```python
from build123d import *

# Parameters (mm, degrees)
F0_W     = 55
F0_H     = 100
F0_R     = 1.55
F0_R_2   = 3.05
F1_DEPTH = 5
F2_SIZE  = 1.5


with BuildPart() as f1:
    # F0 (on Top) → F1 (new body)
    with BuildSketch(Plane.XY):
        with Locations((0, 22.5)):
            Rectangle(F0_W, F0_H)
        with Locations((-20, -22.5)):
            Circle(F0_R, mode=Mode.SUBTRACT)
        with Locations((20, -22.5)):
            Circle(F0_R, mode=Mode.SUBTRACT)
        with Locations((-20, 22.5)):
            Circle(F0_R, mode=Mode.SUBTRACT)
        with Locations((20, 22.5)):
            Circle(F0_R, mode=Mode.SUBTRACT)
        with Locations((0, 52.5)):
            Circle(F0_R_2, mode=Mode.SUBTRACT)
    extrude(amount=F1_DEPTH)

    # F2
    f2_edges = [f1.edges().sort_by_distance(p)[0] for p in [
        (-21.55, 22.5, 5),
        (18.45, 22.5, 5),
        (18.45, -22.5, 5),
        (-21.55, -22.5, 5),
    ]]
    chamfer(f2_edges, length=F2_SIZE)


solid = f1.part
```
Model file for the job. Use its own axes, mm. Coordinates: 2 decimals unless noted, no trailing zeros. Write each loop counter-clockwise with the first axis right and the second up, starting at its lowest first coordinate (ties: lowest second). Pieces come first, ordered by that corner, then holes. Notation, with made-up numbers: (-39.75, 53.5) - (-14.75, 53.5) arc R35 ccw to (-14.75, 92.5) - close; hole circle Ø3 at (3.5, -19.75). An arc over 180 degrees is marked (long way). Use a Markdown table: item, result. Add a question column.
Item 1: Band-saw the part on A-A, the plane x = -20. Write the cut outline in (y, z).
Item 2: Drill centre lines: line 1 along Y through (x, z) = (20, 2.3); line 2 along Y through (x, z) = (0, 3.4); line 3 along Y through (x, z) = (2, 2.55). Where is each one in solid material? Low to high.
Item 3: Band-saw the part on C-C, the plane y = 22.5. Write the cut outline in (x, z).
Item 4: Band-saw the part on B-B, the plane y = 52.5. Write the cut outline in (x, z).
Item 5: Two-plate mould, pull along X, no slides. Class faces 1 (the face through (-0.661, 49.523, 2.465)), 2 (the face through (27.5, 22, 2)), 3 (the face through (0, -27.5, 2)): pulls with the +X half, pulls with the -X half, needs draft (parallel to the pull), parting line crosses it, or undercut.
Item 6: Band-saw the part on D-D, the plane x = 0. Write the cut outline in (y, z).
Item 7: Drop a flat-ended pin along its axis: pin 1 (1.9 mm diameter, centred on x = -20, y = -22.5, fed in from +Z). Give the stop position or say it passes through.
A:
| question | item | result |
|---|---|---|
| 1 | outline | (-27.5, 0) - (-24.05, 0) - (-24.05, 3.5) - (-25.55, 5) - (-27.5, 5) - close; (-20.95, 0) - (20.95, 0) - (20.95, 3.5) - (19.45, 5) - (-19.45, 5) - (-20.95, 3.5) - close; (24.05, 0) - (72.5, 0) - (72.5, 5) - (25.55, 5) - (24.05, 3.5) - close |
| 2 | line 1 | y = -27.5 to -24.05, -20.95 to 20.95, 24.05 to 72.5 |
| 2 | line 2 | y = -27.5 to 49.45, 55.55 to 72.5 |
| 2 | line 3 | y = -27.5 to 50.2, 54.8 to 72.5 |
| 3 | outline | (-27.5, 0) - (-21.55, 0) - (-21.55, 3.5) - (-23.05, 5) - (-27.5, 5) - close; (-18.45, 0) - (18.45, 0) - (18.45, 3.5) - (16.95, 5) - (-16.95, 5) - (-18.45, 3.5) - close; (21.55, 0) - (27.5, 0) - (27.5, 5) - (23.05, 5) - (21.55, 3.5) - close |
| 4 | outline | (-27.5, 0) - (-3.05, 0) - (-3.05, 5) - (-27.5, 5) - close; (3.05, 0) - (27.5, 0) - (27.5, 5) - (3.05, 5) - close |
| 5 | face 1 | undercut |
| 5 | face 2 | pulls with the +X half |
| 5 | face 3 | needs draft |
| 6 | outline | (-27.5, 0) - (49.45, 0) - (49.45, 5) - (-27.5, 5) - close; (55.55, 0) - (72.5, 0) - (72.5, 5) - (55.55, 5) - close |
| 7 | pin 1 | passes through |
